```python
from build123d import *

# Parameters (mm, degrees)
F0_W     = 19.05
F0_H     = 19.05
F0_W_2   = 15.875
F0_H_2   = 15.875
F1_DEPTH = 500
F3_DEPTH = 9.526
F4_DEPTH = 9.526


with BuildPart() as f1:
    # F0 (on Front) → F1 (new body)
    with BuildSketch(Plane.XZ):
        Rectangle(F0_W, F0_H)
        Rectangle(F0_W_2, F0_H_2, mode=Mode.SUBTRACT)
    extrude(amount=F1_DEPTH)

    # F2 (on Top) → F3 (cut, through all)
    with BuildSketch(Plane.XY):
        Polygon((9.525, 0), (-9.525, 0), (-9.525, -19.05), align=None)
        Polygon((-9.525, -480.95), (-9.525, -500), (9.525, -500), align=None)
    extrude(amount=F3_DEPTH, mode=Mode.SUBTRACT)

    # F2 (on Top) → F4 (cut, through all)
    with BuildSketch(Plane.XY):
        Polygon((9.525, 0), (-9.525, 0), (-9.525, -19.05), align=None)
        Polygon((-9.525, -480.95), (-9.525, -500), (9.525, -500), align=None)
    extrude(amount=-F4_DEPTH, mode=Mode.SUBTRACT)


solid = f1.part
```
Read the model definition and answer for the solid it produces. Units are mm, in the model's axes. A direction names the side the tool comes from. Coordinates: 2 decimals unless noted, no trailing zeros. Write each loop counter-clockwise with the first axis right and the second up, starting at its lowest first coordinate (ties: lowest second). Pieces come first, ordered by that corner, then holes. Notation, with made-up numbers: (50.25, 67.25) - (72.25, 67.25) arc R17 cw to (72.25, 93.25) - close; hole circle Ø8 at (-11.75, 8). An arc over 180 degrees is marked (long way). Answer as a JSON object with one key per item and string values. Group by question number.
1. A cutting plane is placed at B-B (x = 1). Determine the outline of the cut face in (y, z) (1 decimal).
2. A cutting plane is placed at C-C (y = -145). Determine the outline of the cut face in (x, z) (1 decimal), plus the area to 3 significant figures.
3. The mould has two halves that part along Z. Classify faces 1 (the flat face through (7.938, -247, 0)), 2 (the flat face through (0, -246, -9.525)), 3 (the flat face through (-7.938, -247, 0)), 4 (the flat face through (0, -246, 9.525)): +Z half, -Z half, draft (parallel to the pull), parting line (faces both ways), or undercut.
4. Consider L1, parallel to X at y = -344.5, z = 6.75 (1 decimal); L2, parallel to Y at x = 8, z = -7.5 (3 decimals). Determine where each line is inside the solid, lowest interval first. Write a range as [from, to].
5. Each of these flat-tipped pins is pushed along its axis until it touches: P1, Ø10, axis at x = -7, z = -4.5, coming from the -Y side; P2, Ø3, axis at x = 3, z = -6, coming from the +Y side. Where does it stop, or does it pass through?
6. Which of the six approach directions +Z, -Z, +X, -X, +Y, -Y give full straight-line access (tool end or side, diameter ignored) to faces 5 (the flat face through (9.525, -246, 0)), 6 (the flat face through (0, -247, 7.938))?
Worked out:
{
 "1": {"outline": "(-491.5, -9.5) - (-8.5, -9.5) - (-8.5, -7.9) - (-491.5, -7.9) - close; (-491.5, 7.9) - (-8.5, 7.9) - (-8.5, 9.5) - (-491.5, 9.5) - close"},
 "2": {"outline": "(-9.5, -9.5) - (9.5, -9.5) - (9.5, 9.5) - (-9.5, 9.5) - close; hole (-7.9, -7.9) - (7.9, -7.9) - (7.9, 7.9) - (-7.9, 7.9) - close", "area": "111 mm²"},
 "3": {"face 1": "undercut", "face 2": "-Z half", "face 3": "undercut", "face 4": "+Z half"},
 "4": {"L1": "x = [-9.5, -7.9], [7.9, 9.5]", "L2": "y = [-498.475, -1.525]"},
 "5": {"P1": "stops at y = -487.11", "P2": "passes through"},
 "6": {"face 5": "+Z, -Z, +X, +Y, -Y", "face 6": "+Y, -Y"}
}
